Design review of the part built by this model. Coordinates are the model's own, in mm. Face numbers are marked on the shaded views. A direction names the side the tool comes from. Give positions to 0.01 mm unless a question says otherwise; leave off trailing zeros. Loops run counter-clockwise (first coordinate to the right, second up) from the corner with the lowest first, then second, coordinate; pieces in that order, holes last. Notation, with made-up numbers: M 42.5,19.5 L 53.5,19.5 A21 ccw 53.5,40.5 Z; hole C -35.5,24 d10. An arc over 180 degrees is marked long. Use a Markdown table: item, result. Add a question column.
(1) Add section C-C, the plane y = -4. Give the boundary of the cut face in (x, z).
(2) For the marked faces 1, 2 and 3, list the 3-axis set-ups (+Z, -Z, +X, -X, +Y, -Y) from which the entire face can be reached by the end or side of a thin tool; tool diameter is ignored.
(3) Insertion check: pin 1 Ø3.5 at (x, y) = (-21.5, -2) entering from +Z; pin 2 Ø3 at (x, z) = (30, 19) entering from -Y; pin 3 Ø15 at (x, z) = (10.5, -14) entering from -Y. Each pin has a flat end and moves straight along its axis. Give the tip position at first contact, or say it passes through.
(4) Add section D-D, the plane z = 13.5. Give the boundary of the cut face in (x, y).
(5) For probe 1 along Z at (x, y) = (14.5, -3.5); probe 2 along Y at (x, z) = (0, -18); probe 3 along X at (y, z) = (-1, 7), list the stretches that pass through material, from the lowest coordinate up.
(6) Add section B-B, the plane z = 5.5. Give the boundary of the cut face in (x, y).
(7) Add section A-A, the plane x = -2. Give the boundary of the cut face in (y, z), then the cut area to 3 significant figures.
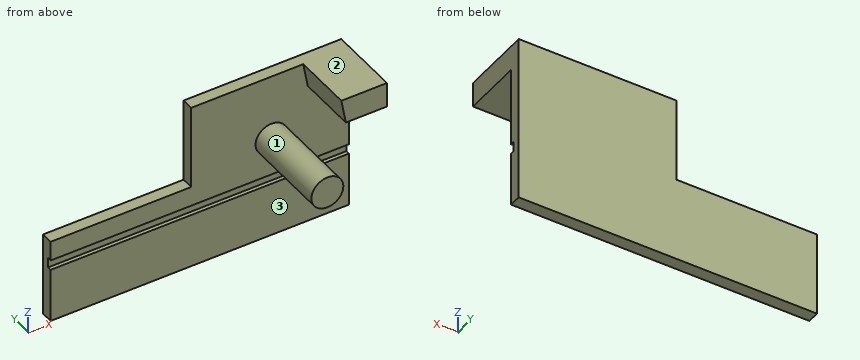
```python
from build123d import *

# Parameters (mm, degrees)
F0_R     = 4
F1_DEPTH = 3
F2_DEPTH = 25
F3_W     = 74.7634656727
F3_H     = 2.5
F4_DEPTH = 1
F5_DEPTH = 18


with BuildPart() as f1:
    # F0 (on Front) → F1 (new body)
    with BuildSketch(Plane.XZ):
        Polygon((-5.3837564774, 0), (-40.6250022352, 0), (-40.6250022352, -21.1607143283), (34.1384634376, -21.1607143283), (34.1384634376, 14.8761495948), (23.8177376958, 14.8761495948), (22.7095993713, 21.1607143283), (-5.3837564774, 21.1607143283), align=None)
        with Locations((14.7321438417, 4.5535718091)):
            Circle(F0_R, mode=Mode.SUBTRACT)
    extrude(amount=F1_DEPTH)

    # F0 (on Front) → F2 (join)
    with BuildSketch(Plane.XZ):
        with Locations((14.7321438417, 4.5535718091)):
            Circle(F0_R)
    extrude(amount=F2_DEPTH)

    # F3 (on face) → F4 (cut)
    with BuildSketch(Plane.XZ.offset(3)):
        with Locations((-3.2432693988, -6.25)):
            Rectangle(F3_W, F3_H)
    extrude(amount=-F4_DEPTH, mode=Mode.SUBTRACT)

    # F0 (on Front) → F5 (join)
    with BuildSketch(Plane.XZ):
        Polygon((23.8177376958, 14.8761495948), (34.1384634376, 14.8761495948), (34.1384634376, 21.1607143283), (22.7095993713, 21.1607143283), align=None)
    extrude(amount=F5_DEPTH)


solid = f1.part
```
Established:
| question | item | result |
|---|---|---|
| 1 | outline | C 14.73,4.55 d8; M 22.71,21.16 L 23.82,14.88 L 34.14,14.88 L 34.14,21.16 Z |
| 2 | face 1 | -Y |
| 2 | face 2 | +Z, +X, -X, +Y, -Y |
| 2 | face 3 | -Z, +X, -X, -Y |
| 3 | pin 1 | z = 0 |
| 3 | pin 2 | y = -18 |
| 3 | pin 3 | y = -3 |
| 4 | outline | M -5.38,-3 L 34.14,-3 L 34.14,0 L -5.38,0 Z |
| 5 | probe 1 | 0.56 to 8.55 |
| 5 | probe 2 | -3 to 0 |
| 5 | probe 3 | -5.38 to 34.14 |
| 6 | outline | M -5.38,-3 L 10.85,-3 L 10.85,-25 L 18.62,-25 L 18.62,-3 L 34.14,-3 L 34.14,0 L -5.38,0 Z |
| 7 | outline | M -3,-21.16 L 0,-21.16 L 0,21.16 L -3,21.16 L -3,-5 L -2,-5 L -2,-7.5 L -3,-7.5 Z |
| 7 | area | 124 mm^2 |
